```python
from build123d import *

# Parameters (mm, degrees)
F0_W     = 31.75
F0_H     = 60.198
F0_R     = 7.874
F1_DEPTH = 10.922
F3_DEPTH = 10.922
F2_W     = 10.922
F2_H     = 33.528
F4_DEPTH = 22.098
F6_DEPTH = 10.922


with BuildPart() as f1:
    # F0 (on Front) → F1 (new body)
    with BuildSketch(Plane.XZ):
        Rectangle(F0_W, F0_H)
        Polygon((111.125, 4.576839), (15.875, 30.099), (15.875, -30.099), (111.125, -30.099), align=None)
        with Locations((92.075, -11.049)):
            Circle(F0_R, mode=Mode.SUBTRACT)
    extrude(amount=F1_DEPTH)

    # F2 (on face) → F3 (join)
    with BuildSketch(Plane(origin=(0, 0, -30.099), x_dir=(1, 0, 0), z_dir=(0, 0, -1))):
        Polygon((-4.953, 44.45), (-4.953, 10.922), (47.625, 10.922), align=None)
    extrude(amount=-F3_DEPTH)

    # F2 (on face) → F4 (join)
    with BuildSketch(Plane(origin=(0, 0, -30.099), x_dir=(1, 0, 0), z_dir=(0, 0, -1))):
        with Locations((-10.414, 27.686)):
            Rectangle(F2_W, F2_H)
    extrude(amount=-F4_DEPTH)

    # F5 (on face) → F6 (join)
    with BuildSketch(Plane(origin=(-15.875, 0, 0), x_dir=(0, -1, 0), z_dir=(-1, 0, 0))):
        Polygon((10.922, -8.001), (44.45, -8.001), (27.878893, 20.701), (10.922, 20.701), align=None)
    extrude(amount=-F6_DEPTH)


solid = f1.part
```
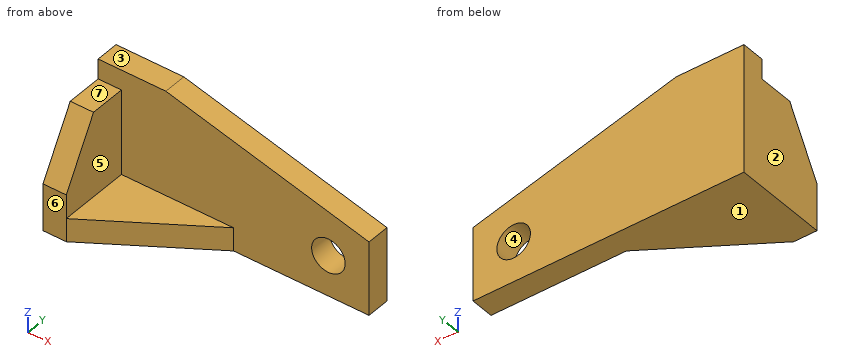
Geometry check sheet. Reference: the model listing, model coordinates, mm. Face numbers are marked on the shaded views. A direction names the side the tool comes from. Give positions to 0.01 mm unless a question says otherwise; leave off trailing zeros. Write each loop counter-clockwise with the first axis right and the second up, starting at its lowest first coordinate (ties: lowest second). Pieces come first, ordered by that corner, then holes.
1) Release check for a two-part mould opening along Z. For the marked faces 1, 2, 3 and 4 record: pulls with the +Z half, pulls with the -Z half, needs draft (parallel to the pull), parting line crosses it, or undercut.
2) Access from +Z, -Z, +X, -X, +Y, -Y to the whole of each face (thin tool, end or side, straight path). Record for the marked faces 5, 6 and 7.
3) Gauge pin test, flat ends, axial feed: pin 1 (4 mm diameter, centred on y = -23.5, z = -19, fed in from +X); pin 2 (10 mm diameter, centred on x = 22, y = -24.5, fed in from +Z); pin 3 (12 mm diameter, centred on y = -17.5, z = 2.5, fed in from +X); pin 4 (6 mm diameter, centred on x = 17, z = 2.5, fed in from +Y). Record the tip position at first contact, or that the pin passes through.
4) Material ranges on L1, parallel to Z at x = 15, y = -21; L2, parallel to Y at x = 19.5, z = 2.5; L3, parallel to X at y = -2.5, z = -10.5 (3 decimals), recorded low to high.
5) Section check A-A, the plane x = 98.5. Record the boundary of the cut face in (y, z), and give its area (3 significant figures).
6) Section check D-D, the plane y = -40. Record the boundary of the cut face in (x, z) (3 decimals), and give its area (3 significant figures).
7) Section check B-B, the plane z = -25. Record the boundary of the cut face in (x, y) (3 decimals), and give its area (3 significant figures).
8) Section check C-C, the plane y = -4.5. Record the boundary of the cut face in (x, z) (3 decimals), and give its area (3 significant figures).
Computed:
1. face 1: pulls with the -Z half
1. face 2: needs draft
1. face 3: pulls with the +Z half
1. face 4: undercut
2. face 5: +Z, +X, -Y
2. face 6: +Z, -Z, +X, -X, -Y
2. face 7: +Z, +X, -X, -Y
3. pin 1: stops at x = 31.02
3. pin 2: stops at z = -19.18
3. pin 3: stops at x = -4.95
3. pin 4: stops at y = 0
4. L1: z = -30.1 to -19.18
4. L2: y = -10.92 to 0
4. L3: x = -15.875 to 84.22, 99.93 to 111.125
5. outline: (-10.92, -30.1) - (0, -30.1) - (0, -15.6) - (-10.92, -15.6) - close; (-10.92, -6.5) - (0, -6.5) - (0, 7.96) - (-10.92, 7.96) - close
5. area: 316 mm2
6. outline: (-15.875, -30.099) - (2.025, -30.099) - (2.025, -19.177) - (-4.953, -19.177) - (-4.953, -0.293) - (-15.875, -0.293) - close
6. area: 402 mm2
7. outline: (-15.875, -44.45) - (-4.953, -44.45) - (47.625, -10.922) - (111.125, -10.922) - (111.125, 0) - (-15.875, 0) - close
7. area: 2,630 mm2
8. outline: (-15.875, -30.099) - (111.125, -30.099) - (111.125, 4.577) - (15.875, 30.099) - (-15.875, 30.099) - close; hole circle Ø15.748 at (92.075, -11.049)
8. area: 6,230 mm2
